Check sheet for the drawn part. Datum: minimum x, y, z corner. Units: mm. Give positions to 0.01 mm unless a question says otherwise; leave off trailing zeros. Write each loop counter-clockwise with the first axis right and the second up, starting at its lowest first coordinate (ties: lowest second). Pieces come first, ordered by that corner, then holes. Notation, with made-up numbers: (-15, 74) -> (-4, 74) arc R25 ccw to (-4, 109) -> close; hole circle Ø2 at (-36, -4.75). An arc over 180 degrees is marked (long way). Use CSV: the item, a comma, the result in double quotes. Start each with the question number.
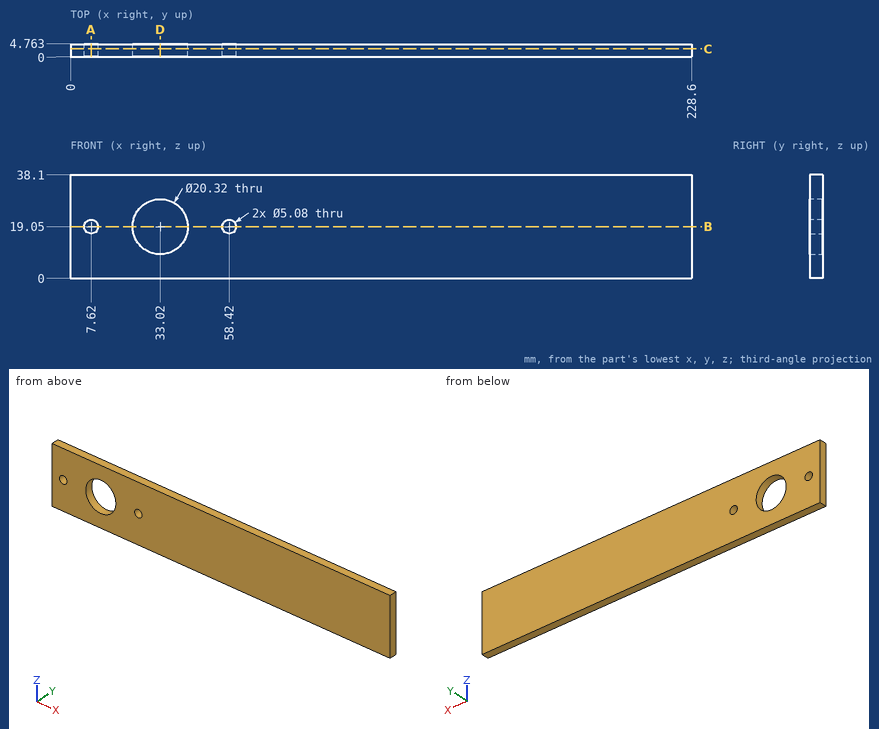
(1) Section check D-D on x = 33.02. Record the cut outline in (y, z).
(2) Section check B-B on z = 19.05. Record the cut outline in (x, y).
(3) Thickness scan on line 1 (X direction, y = 2.95, z = 19.05); line 2 (Z direction, x = 58.42, y = 3.5); line 3 (X direction, y = 1.8, z = 17). Record the ranges inside material, lowest first. Write a range as from..to.
(4) Section check A-A on x = 7.62. Record the cut outline in (y, z).
(5) Section check C-C on y = 3. Record the cut outline in (x, z).
Data:
1,outline,"(0, 0) -> (4.76, 0) -> (4.76, 8.89) -> (0, 8.89) -> close; (0, 29.21) -> (4.76, 29.21) -> (4.76, 38.1) -> (0, 38.1) -> close"
2,outline,"(0, 0) -> (5.08, 0) -> (5.08, 4.76) -> (0, 4.76) -> close; (10.16, 0) -> (22.86, 0) -> (22.86, 4.76) -> (10.16, 4.76) -> close; (43.18, 0) -> (55.88, 0) -> (55.88, 4.76) -> (43.18, 4.76) -> close; (60.96, 0) -> (228.6, 0) -> (228.6, 4.76) -> (60.96, 4.76) -> close"
3,line 1,"x = 0..5.08, 10.16..22.86, 43.18..55.88, 60.96..228.6"
3,line 2,"z = 0..16.51, 21.59..38.1"
3,line 3,"x = 0..6.12, 9.12..23.07, 42.97..56.92, 59.92..228.6"
4,outline,"(0, 0) -> (4.76, 0) -> (4.76, 16.51) -> (0, 16.51) -> close; (0, 21.59) -> (4.76, 21.59) -> (4.76, 38.1) -> (0, 38.1) -> close"
5,outline,"(0, 0) -> (228.6, 0) -> (228.6, 38.1) -> (0, 38.1) -> close; hole circle Ø5.08 at (7.62, 19.05); hole circle Ø20.32 at (33.02, 19.05); hole circle Ø5.08 at (58.42, 19.05)"
